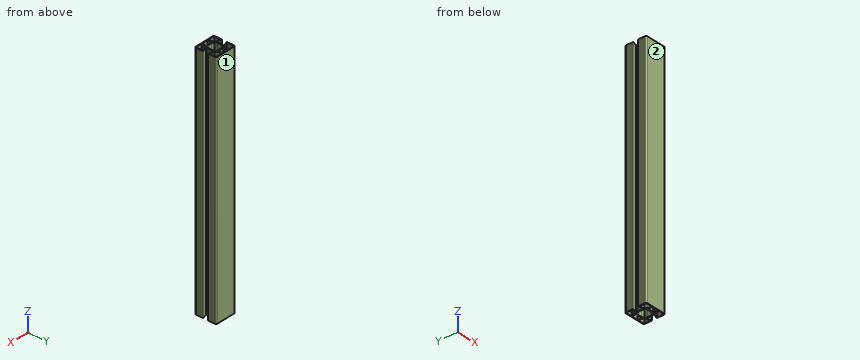
from build123d import *

# Parameters (mm, degrees)
F1_DEPTH = 1000


# Not quite as in the source:
# - ends of sketch curves that miss each other by under 0.0002 mm in the source are joined


with BuildPart() as f1:
    # F0 (on Top) → F1 (new body)
    with BuildSketch(Plane.XY):
        with BuildLine():
            ThreePointArc((23.0888885991, 8.8614578186), (23.022474706, 9.062799833), (23, 9.273618))
            Line((23, 9.273618), (23, 14.841657))
            ThreePointArc((23, 14.841657), (23.3912385359, 15.6350103133), (24.2588189596, 15.8075828492))
            Line((24.2588189596, 15.8075828492), (43.426476, 10.671624))
            ThreePointArc((43.426476, 10.671624), (44.5109517857, 10.8873403242), (45, 11.879032))
            Line((45, 11.879032), (45, 39))
            ThreePointArc((45, 39), (43.2426406871, 43.2426406871), (39, 45))
            Line((39, 45), (-39, 45))
            ThreePointArc((-39, 45), (-43.2426406871, 43.2426406871), (-45, 39))
            Line((-45, 39), (-45, 11.879032))
            ThreePointArc((-45, 11.879032), (-44.5109517857, 10.8873403242), (-43.4264761923, 10.6716247175))
            Line((-43.4264761923, 10.6716247175), (-24.258819, 15.807583))
            ThreePointArc((-24.258819, 15.807583), (-23.3912385359, 15.6350103133), (-23, 14.841657))
            Line((-23, 14.841657), (-23, 9.273618))
            ThreePointArc((-23, 9.273618), (-23.022474706, 9.062799833), (-23.0888885991, 8.8614578186))
            ThreePointArc((-23.0888885991, 8.8614578186), (-25, 0), (-23.0888887851, -8.8614579028))
            ThreePointArc((-23.0888887851, -8.8614579028), (-23.022474706, -9.062799833), (-23, -9.273618))
            Line((-23, -9.273618), (-23, -14.841657))
            ThreePointArc((-23, -14.841657), (-23.3912385359, -15.6350103133), (-24.2588189596, -15.8075828492))
            Line((-24.2588189596, -15.8075828492), (-43.426476, -10.671624))
            ThreePointArc((-43.426476, -10.671624), (-44.5109517857, -10.8873403242), (-45, -11.879032))
            Line((-45, -11.879032), (-45, -39))
            ThreePointArc((-45, -39), (-43.2426406871, -43.2426406871), (-39, -45))
            Line((-39, -45), (39, -45))
            ThreePointArc((39, -45), (43.2426406871, -43.2426406871), (45, -39))
            Line((45, -39), (45, -11.879032))
            ThreePointArc((45, -11.879032), (44.5109517857, -10.8873403242), (43.4264761923, -10.6716247175))
            Line((43.4264761923, -10.6716247175), (24.258819, -15.807583))
            ThreePointArc((24.258819, -15.807583), (23.3912385359, -15.6350103133), (23, -14.841657))
            Line((23, -14.841657), (23, -9.273618))
            ThreePointArc((23, -9.273618), (23.022474706, -9.062799833), (23.0888885991, -8.8614578186))
            ThreePointArc((23.0888885991, -8.8614578186), (25, 0), (23.0888885991, 8.8614578186))
        make_face()
        with BuildLine():
            Line((-14.841657, -23), (-9.273618, -23))
            ThreePointArc((-9.273618, -23), (-9.062799833, -23.022474706), (-8.8614578186, -23.0888885991))
            ThreePointArc((-8.8614578186, -23.0888885991), (0, -25), (8.8614579028, -23.0888887851))
            ThreePointArc((8.8614579028, -23.0888887851), (9.062799833, -23.022474706), (9.273618, -23))
            Line((9.273618, -23), (14.841657, -23))
            ThreePointArc((14.841657, -23), (15.6350103133, -23.3912385359), (15.8075828492, -24.2588189596))
            Line((15.8075828492, -24.2588189596), (10.98686, -42.25))
            Line((10.98686, -42.25), (-10.98686, -42.25))
            Line((-10.98686, -42.25), (-15.807583, -24.258819))
            ThreePointArc((-15.807583, -24.258819), (-15.6350103133, -23.3912385359), (-14.841657, -23))
        make_face(mode=Mode.SUBTRACT)
        with BuildLine():
            Line((-39.732362, -14.508469), (-24.482362, -18.594694))
            ThreePointArc((-24.482362, -18.594694), (-23.4132933733, -19.3090230718), (-23, -20.526546))
            Line((-23, -20.526546), (-23, -21))
            ThreePointArc((-23, -21), (-22.4142135624, -22.4142135624), (-21, -23))
            Line((-21, -23), (-20.526546, -23))
            ThreePointArc((-20.526546, -23), (-19.3090230718, -23.4132933733), (-18.5946943016, -24.4823620808))
            Line((-18.5946943016, -24.4823620808), (-14.508469, -39.732362))
            ThreePointArc((-14.508469, -39.732362), (-14.8536143733, -41.4675229282), (-16.440321, -42.25))
            Line((-16.440321, -42.25), (-39, -42.25))
            ThreePointArc((-39, -42.25), (-41.2980970389, -41.2980970389), (-42.25, -39))
            Line((-42.25, -39), (-42.25, -16.440321))
            ThreePointArc((-42.25, -16.440321), (-41.4675229282, -14.8536143733), (-39.732362, -14.508469))
        make_face(mode=Mode.SUBTRACT)
        with BuildLine():
            Line((14.508469, -39.732362), (18.594694, -24.482362))
            ThreePointArc((18.594694, -24.482362), (19.3090230718, -23.4132933733), (20.526546, -23))
            Line((20.526546, -23), (21, -23))
            ThreePointArc((21, -23), (22.4142135624, -22.4142135624), (23, -21))
            Line((23, -21), (23, -20.526546))
            ThreePointArc((23, -20.526546), (23.4132933733, -19.3090230718), (24.4823620808, -18.5946943016))
            Line((24.4823620808, -18.5946943016), (39.732362, -14.508469))
            ThreePointArc((39.732362, -14.508469), (41.4675229282, -14.8536143733), (42.25, -16.440321))
            Line((42.25, -16.440321), (42.25, -39))
            ThreePointArc((42.25, -39), (41.2980970389, -41.2980970389), (39, -42.25))
            Line((39, -42.25), (16.440321, -42.25))
            ThreePointArc((16.440321, -42.25), (14.8536143733, -41.4675229282), (14.508469, -39.732362))
        make_face(mode=Mode.SUBTRACT)
        with BuildLine():
            Line((-7.3951, -20.25), (-19.25, -20.25))
            ThreePointArc((-19.25, -20.25), (-19.9571067812, -19.9571067812), (-20.25, -19.25))
            Line((-20.25, -19.25), (-20.25, -7.3951))
            ThreePointArc((-20.25, -7.3951), (-20.2639867072, -7.2284333074), (-20.3055555728, -7.0664288513))
            ThreePointArc((-20.3055554887, -7.066428822), (-21.5, 0), (-20.3055554887, 7.066428822))
            ThreePointArc((-20.3055555728, 7.0664288513), (-20.2639867072, 7.2284333074), (-20.25, 7.3951))
            Line((-20.25, 7.3951), (-20.25, 19.25))
            ThreePointArc((-20.25, 19.25), (-19.9571067812, 19.9571067812), (-19.25, 20.25))
            Line((-19.25, 20.25), (-7.3951, 20.25))
            ThreePointArc((-7.3951, 20.25), (-7.2284333074, 20.2639867072), (-7.0664288513, 20.3055555728))
            ThreePointArc((-7.066428822, 20.3055554887), (0, 21.5), (7.066428822, 20.3055554887))
            ThreePointArc((7.0664288513, 20.3055555728), (7.2284333074, 20.2639867072), (7.3951, 20.25))
            Line((7.3951, 20.25), (19.25, 20.25))
            ThreePointArc((19.25, 20.25), (19.9571067812, 19.9571067812), (20.25, 19.25))
            Line((20.25, 19.25), (20.25, 7.3951))
            ThreePointArc((20.25, 7.3951), (20.2639867072, 7.2284333074), (20.3055555728, 7.0664288513))
            ThreePointArc((20.3055554887, 7.066428822), (21.5, 0), (20.3055554887, -7.066428822))
            ThreePointArc((20.3055555728, -7.0664288513), (20.2639867072, -7.2284333074), (20.25, -7.3951))
            Line((20.25, -7.3951), (20.25, -19.25))
            ThreePointArc((20.25, -19.25), (19.9571067812, -19.9571067812), (19.25, -20.25))
            Line((19.25, -20.25), (7.3951, -20.25))
            ThreePointArc((7.3951, -20.25), (7.2284333074, -20.2639867072), (7.0664288513, -20.3055555728))
            ThreePointArc((7.066428822, -20.3055554887), (0, -21.5), (-7.066428822, -20.3055554887))
            ThreePointArc((-7.0664288513, -20.3055555728), (-7.2284333074, -20.2639867072), (-7.3951, -20.25))
        make_face(mode=Mode.SUBTRACT)
        with BuildLine():
            Line((-14.508469, 39.732362), (-18.594694, 24.482362))
            ThreePointArc((-18.594694, 24.482362), (-19.3090230718, 23.4132933733), (-20.526546, 23))
            Line((-20.526546, 23), (-21, 23))
            ThreePointArc((-21, 23), (-22.4142135624, 22.4142135624), (-23, 21))
            Line((-23, 21), (-23, 20.526546))
            ThreePointArc((-23, 20.526546), (-23.4132933733, 19.3090230718), (-24.4823620808, 18.5946943016))
            Line((-24.4823620808, 18.5946943016), (-39.732362, 14.508469))
            ThreePointArc((-39.732362, 14.508469), (-41.4675229282, 14.8536143733), (-42.25, 16.440321))
            Line((-42.25, 16.440321), (-42.25, 39))
            ThreePointArc((-42.25, 39), (-41.2980970389, 41.2980970389), (-39, 42.25))
            Line((-39, 42.25), (-16.440321, 42.25))
            ThreePointArc((-16.440321, 42.25), (-14.8536143733, 41.4675229282), (-14.508469, 39.732362))
        make_face(mode=Mode.SUBTRACT)
        with BuildLine():
            Line((-15.807583, 24.258819), (-10.98686, 42.25))
            Line((-10.98686, 42.25), (10.98686, 42.25))
            Line((10.98686, 42.25), (15.807583, 24.258819))
            ThreePointArc((15.807583, 24.258819), (15.6350103133, 23.3912385359), (14.841657, 23))
            Line((14.841657, 23), (9.273618, 23))
            ThreePointArc((9.273618, 23), (9.062799833, 23.022474706), (8.8614578186, 23.0888885991))
            ThreePointArc((8.8614578186, 23.0888885991), (0, 25), (-8.8614579028, 23.0888887851))
            ThreePointArc((-8.8614579028, 23.0888887851), (-9.062799833, 23.022474706), (-9.273618, 23))
            Line((-9.273618, 23), (-14.841657, 23))
            ThreePointArc((-14.841657, 23), (-15.6350103133, 23.3912385359), (-15.807583, 24.258819))
        make_face(mode=Mode.SUBTRACT)
        with BuildLine():
            Line((39.732362, 14.508469), (24.482362, 18.594694))
            ThreePointArc((24.482362, 18.594694), (23.4132933733, 19.3090230718), (23, 20.526546))
            Line((23, 20.526546), (23, 21))
            ThreePointArc((23, 21), (22.4142135624, 22.4142135624), (21, 23))
            Line((21, 23), (20.526546, 23))
            ThreePointArc((20.526546, 23), (19.3090230718, 23.4132933733), (18.5946943016, 24.4823620808))
            Line((18.5946943016, 24.4823620808), (14.508469, 39.732362))
            ThreePointArc((14.508469, 39.732362), (14.8536143733, 41.4675229282), (16.440321, 42.25))
            Line((16.440321, 42.25), (39, 42.25))
            ThreePointArc((39, 42.25), (41.2980970389, 41.2980970389), (42.25, 39))
            Line((42.25, 39), (42.25, 16.440321))
            ThreePointArc((42.25, 16.440321), (41.4675229282, 14.8536143733), (39.732362, 14.508469))
        make_face(mode=Mode.SUBTRACT)
    extrude(amount=F1_DEPTH)


solid = f1.part
Could you check a few things on this model? Use its own coordinates, in mm. Face numbers are marked on the shaded views. Give positions to 0.01 mm unless a question says otherwise; leave off trailing zeros. One line per item, written item: value. Start each with the question number.
1. Thinking about a two-plate mould opening in Y: for the marked faces 1 and 2, which applies, +Y half, -Y half, draft (parallel to the pull), parting line (faces both ways), or undercut?
2. For P1, Ø6, axis at y = 0, z = 560.5, coming from the +X side; P2, Ø6, axis at y = -11.5, z = 585.5, coming from the +X side; P3, Ø2, axis at y = 10.5, z = 362.5, coming from the +X side, each with a flat end and sliding along its axis, tell me the tip position at first contact or that it passes through.
3. If I drill on probe 1 along Y at (x, z) = (39.5, 48); probe 2 along Y at (x, z) = (10.5, 879); probe 3 along X at (y, z) = (38.5, 920), over which ranges is the centre line in solid material (lowest first)?
4. Imagine slicing it at A-A on z = 620. Give the number of separate pieces and of enclosed holes in the cut face, plus the area to 3 significant figures.
Values:
1. face 1: +Y half
1. face 2: -Y half
2. P1: x = 25
2. P2: x = 45
2. P3: x = 44.94
3. probe 1: -44.98 to -42.21, -14.57 to -11.72, 11.72 to 14.57, 42.21 to 44.98
3. probe 2: -45 to -42.25, -23 to -20.25, 20.25 to 23, 42.25 to 45
3. probe 3: -45 to -42.25, -14.84 to -11.99, 11.99 to 14.84, 42.25 to 45
4. separate pieces: 1
4. enclosed holes: 7
4. area: 1,800 mm²
